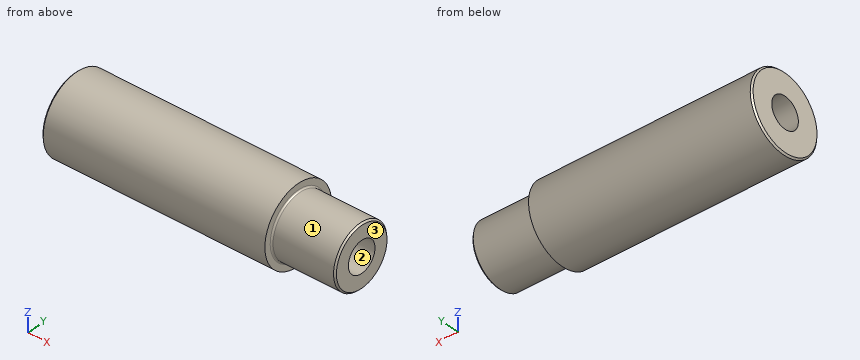
from build123d import *

# Parameters (mm, degrees)
SKETCH1_R           = 12.5
SKETCH1_R_2         = 5
BOSS_EXTRUDE1_DEPTH = 92.5
SKETCH2_OUTSIDE_W   = 46.806
SKETCH2_OUTSIDE_H   = 46.806
SKETCH2_OUTSIDE_R   = 10
CUT_EXTRUDE1_DEPTH  = 20.5
FILLET1_R           = 0.5
CHAMFER1_SIZE       = 0.5


with BuildPart() as part:
    # Sketch1 → Boss-Extrude1 (new body)
    with BuildSketch(Plane(origin=(0, 0, 0), x_dir=(0, 0, -1), z_dir=(1, 0, 0))):
        Circle(SKETCH1_R)
        Circle(SKETCH1_R_2, mode=Mode.SUBTRACT)
    extrude(amount=BOSS_EXTRUDE1_DEPTH)

    # Sketch2 outside → Cut-Extrude1 (cut)
    with BuildSketch(Plane(origin=(92.5, 0, 0), x_dir=(0, 0, -1), z_dir=(1, 0, 0))):
        Rectangle(SKETCH2_OUTSIDE_W, SKETCH2_OUTSIDE_H)
        Circle(SKETCH2_OUTSIDE_R, mode=Mode.SUBTRACT)
    extrude(amount=-CUT_EXTRUDE1_DEPTH, mode=Mode.SUBTRACT)

    # Fillet1
    fillet1_edges = [part.edges().sort_by_distance(p)[0] for p in [
        (72, 0, 10),
    ]]
    fillet(fillet1_edges, radius=FILLET1_R)

    # Chamfer1
    chamfer1_edges = [part.edges().sort_by_distance(p)[0] for p in [
        (92.5, 0, 10),
        (0, 0, 12.5),
    ]]
    chamfer(chamfer1_edges, length=CHAMFER1_SIZE)


solid = part.part
Can you work these out from the model? Positions are in its coordinate system, mm. Face numbers are marked on the shaded views. Give positions to 0.01 mm unless a question says otherwise; leave off trailing zeros. Write each loop counter-clockwise with the first axis right and the second up, starting at its lowest first coordinate (ties: lowest second). Pieces come first, ordered by that corner, then holes. Notation, with made-up numbers: M -37,69.5 L 18,69.5 A16 ccw 18,74.5 Z; hole C -39.75,-31 d2. An arc over 180 degrees is marked long. Answer in a Markdown table with one row per item. Add a question column.
Item 1: We'd pull the mould along Y, two halves only. Please class the marked faces 1, 2 and 3: released by +Y, released by -Y, zero draft, split by the parting line, or undercut.
Item 2: Imagine slicing it at C-C, the plane x = 82. Write out the boundary of the cut face in (y, z).
Item 3: For pin 1 Ø6 at (x, y) = (11, 9.5) entering from -Z; pin 2 Ø1.5 at (x, y) = (43, 4.5) entering from +Z; pin 3 Ø5 at (x, z) = (33.5, -0.5) entering from +Y; pin 4 Ø5 at (x, z) = (24.5, -9.5) entering from -Y, each with a flat end and sliding along its axis, tell me the tip position at first contact or that it passes through.
Item 4: Imagine slicing it at D-D, the plane x = 34. Write out the boundary of the cut face in (y, z).
Item 5: Imagine slicing it at A-A, the plane y = 0. Write out the boundary of the cut face in (x, z), plus the area to 3 significant figures.
Item 6: Please list where these lines run through material, in increasing order: L1, parallel to Z at x = 55, y = -0.25; L2, parallel to Y at x = 52, z = 0; L3, parallel to Y at x = 76, z = -3.5.
Evaluation:
| question | item | result |
|---|---|---|
| 1 | face 1 | split by the parting line |
| 1 | face 2 | undercut |
| 1 | face 3 | zero draft |
| 2 | outline | C 0,0 d20; hole C 0,0 d10 |
| 3 | pin 1 | stops at z = -10.68 |
| 3 | pin 2 | stops at z = 11.92 |
| 3 | pin 3 | stops at y = 12.5 |
| 3 | pin 4 | stops at y = -10.36 |
| 4 | outline | C 0,0 d25; hole C 0,0 d10 |
| 5 | outline | M 0,-12 L 0.5,-12.5 L 72,-12.5 L 72,-10.5 A0.5 cw 72.5,-10 L 92,-10 L 92.5,-9.5 L 92.5,-5 L 0,-5 Z; M 0,5 L 92.5,5 L 92.5,9.5 L 92,10 L 72.5,10 A0.5 cw 72,10.5 L 72,12.5 L 0.5,12.5 L 0,12 Z |
| 5 | area | 1,280 mm² |
| 6 | L1 | z = -12.5 to -4.99, 4.99 to 12.5 |
| 6 | L2 | y = -12.5 to -5, 5 to 12.5 |
| 6 | L3 | y = -9.37 to -3.57, 3.57 to 9.37 |
